```python
from build123d import *

# Parameters (mm, degrees)
EXTRUDE_1_DEPTH   = 2.4
HOLE_WIZARD_M31_D = 2.5
CHAMFER_1_SIZE    = 0.5


with BuildPart() as part:
    # Эскиз1 → Бобышка-Вытянуть1 (new body)
    with BuildSketch(Plane.XY):
        Polygon((2.75, 1.58771324), (0, 3.175426481), (-2.75, 1.58771324), (-2.75, -1.58771324), (0, -3.175426481), (2.75, -1.58771324), align=None)
    extrude(amount=EXTRUDE_1_DEPTH)

    # Отверстие обработанное метчиком M31 (through all)
    with Locations(Plane.XY.offset(2.4)):
        with Locations((0, 0)):
            Hole(HOLE_WIZARD_M31_D / 2)

    # Фаска1
    chamfer_1_edges = [part.edges().sort_by_distance(p)[0] for p in [
        (1.25, 0, 2.4),
        (1.25, 0, 0),
    ]]
    chamfer(chamfer_1_edges, length=CHAMFER_1_SIZE)

    # Эскиз4 → Вырез-Повернуть1 (revolve, cut)
    with BuildSketch(Plane(origin=(0, 0, 0), x_dir=(0, 0, -1), z_dir=(1, 0, 0)), mode=Mode.PRIVATE) as cut_revolve_1_sk:
        Polygon((0, 2.75), (0, 4), (-0.721687836, 4), align=None)
        Polygon((-2.4, 2.75), (-2.4, 4), (-1.678312164, 4), align=None)
    revolve(cut_revolve_1_sk.sketch.rotate(Axis((0, 0, 0), (0, 0, 1)), 270), axis=Axis((0, 0, 0), (0, 0, 1)), mode=Mode.SUBTRACT)


solid = part.part
```
Model file for the job. Use its own axes, mm. Coordinates: 2 decimals unless noted, no trailing zeros. Order: outer loops, then holes, each group sorted by start corner. A loop starts at its lowest first (then second) coordinate and runs counter-clockwise, first axis right, second up. Notation, with made-up numbers: (-23.5, 18.25) -> (32.5, 18.25) arc R38 ccw to (32.5, 57.25) -> close; hole circle Ø5 at (52.25, 33). An arc over 180 degrees is marked (long way). Return JSON: item names as keys, results as strings.
Item 1: Pin check, flat tip, straight feed: P1, Ø3, axis at x = 0, y = 0, coming from the -Z side. Stop position of the tip, or through.
Model answer:
{"P1": "stops at z = 0.25"}
Item 2: Slice it at A-A (z = 0.4). Write the cut outline in (x, y).
Model answer:
{"outline": "(-2.75, -1.59) -> (0, -3.18) -> (2.75, -1.59) -> (2.75, 1.59) -> (0, 3.18) -> (-2.75, 1.59) -> close; hole circle Ø2.7 at (0, 0)"}
Item 3: Wall check: line 1 along X through (y, z) = (-0.25, 2.1); line 2 along Y through (x, z) = (1, 1.05); line 3 along X through (y, z) = (0.5, 1.1). Give the ranges that are in metal, low to high. Write a range as from..to.
Model answer:
{"line 1": "x = -2.75..-1.43, 1.43..2.75", "line 2": "y = -2.6..-0.75, 0.75..2.6", "line 3": "x = -2.75..-1.15, 1.15..2.75"}
Item 4: Slice it at B-B (z = 2.05). Write the cut outline in (x, y).
Model answer:
{"outline": "(-2.75, -1.59) -> (0, -3.18) -> (2.75, -1.59) -> (2.75, 1.59) -> (0, 3.18) -> (-2.75, 1.59) -> close; hole circle Ø2.8 at (0, 0)"}
